from build123d import *

# Parameters (mm, degrees)
SKETCH1_W           = 70
SKETCH1_H           = 40
BOSS_EXTRUDE1_DEPTH = 1.7
SKETCH2_R           = 1
CUT_EXTRUDE1_DEPTH  = 1.7
SKETCH3_R           = 14
BOSS_EXTRUDE2_DEPTH = 30
SKETCH4_W           = 9.678505403
SKETCH4_H           = 8
BOSS_EXTRUDE3_DEPTH = 4
SKETCH5_W           = 6
SKETCH5_H           = 3
BOSS_EXTRUDE4_DEPTH = 4
SKETCH6_W           = 62
SKETCH6_H           = 32
BOSS_EXTRUDE5_DEPTH = 1
SKETCH7_W           = 35.794081109
SKETCH7_H           = 31.717706103
BOSS_EXTRUDE6_DEPTH = 1


with BuildPart() as part:
    # Sketch1 → Boss-Extrude1 (new body)
    with BuildSketch(Plane(origin=(0, 0, 0), x_dir=(1, 0, 0), z_dir=(0, 1, 0))):
        with Locations((35, 20)):
            Rectangle(SKETCH1_W, SKETCH1_H)
    extrude(amount=BOSS_EXTRUDE1_DEPTH)

    # Sketch2 → Cut-Extrude1 (cut)
    with BuildSketch(Plane(origin=(0, 1.7, 0), x_dir=(1, 0, 0), z_dir=(0, 1, 0))):
        with Locations(Location((67.8, 37.8, 0), (0, 0, 270))):
            Circle(SKETCH2_R)
        with Locations(Location((2.2, 37.8, 0), (0, 0, 270))):
            Circle(SKETCH2_R)
        with Locations(Location((2.2, 2.2, 0), (0, 0, 270))):
            Circle(SKETCH2_R)
        with Locations(Location((67.8, 2.2, 0), (0, 0, 270))):
            Circle(SKETCH2_R)
    extrude(amount=-CUT_EXTRUDE1_DEPTH, mode=Mode.SUBTRACT)

    # Sketch3 → Boss-Extrude2 (add)
    with BuildSketch(Plane(origin=(0, 1.7, 0), x_dir=(1, 0, 0), z_dir=(0, 1, 0))):
        with Locations(Location((15, 20, 0), (0, 0, 90))):
            Circle(SKETCH3_R)
    extrude(amount=BOSS_EXTRUDE2_DEPTH)

    # Sketch4 → Boss-Extrude3 (add)
    with BuildSketch(Plane(origin=(0, 1.7, 0), x_dir=(1, 0, 0), z_dir=(0, 1, 0))):
        with Locations((65.160747298, 27)):
            Rectangle(SKETCH4_W, SKETCH4_H)
    extrude(amount=BOSS_EXTRUDE3_DEPTH)

    # Sketch5 → Boss-Extrude4 (add)
    with BuildSketch(Plane(origin=(0, 1.7, 0), x_dir=(1, 0, 0), z_dir=(0, 1, 0))):
        with Locations((57, 16.5)):
            Rectangle(SKETCH5_W, SKETCH5_H)
    extrude(amount=BOSS_EXTRUDE4_DEPTH)

    # Sketch6 → Boss-Extrude5 (add)
    with BuildSketch(Plane.XZ):
        with Locations((35, -20)):
            Rectangle(SKETCH6_W, SKETCH6_H)
    extrude(amount=BOSS_EXTRUDE5_DEPTH)

    # Sketch7 → Boss-Extrude6 (add)
    with BuildSketch(Plane(origin=(0, 1.7, 0), x_dir=(1, 0, 0), z_dir=(0, 1, 0))):
        with Locations((48.346916126, 21.020495195)):
            Rectangle(SKETCH7_W, SKETCH7_H)
    extrude(amount=BOSS_EXTRUDE6_DEPTH)


solid = part.part
Could you check a few things on this model? Use its own coordinates, in mm. A direction names the side the tool comes from. Coordinates: 2 decimals unless noted, no trailing zeros. Write each loop counter-clockwise with the first axis right and the second up, starting at its lowest first coordinate (ties: lowest second). Pieces come first, ordered by that corner, then holes. Notation, with made-up numbers: (3.5, 71.5) - (10.5, 71.5) arc R36 cw to (10.5, 106.5) - close; hole circle Ø6 at (70, -16). An arc over 180 degrees is marked (long way). Put each result on its own line as item: value. Start each with the question number.
Q1. I want a section at B-B on x = 67.8. Write out the boundary of the cut face in (y, z), plus the area to 3 significant figures.
Q2. I want a section at D-D on z = -20. Write out the boundary of the cut face in (x, y), plus the area to 3 significant figures.
Q3. I want a section at A-A on z = -37.8. Write out the boundary of the cut face in (x, y).
Q4. I want a section at C-C on x = 15. Write out the boundary of the cut face in (y, z), plus the area to 3 significant figures.
Q5. Which directions (+Z, -Z, +X, -X, +Y, -Y) give clear straight access to the entire face, cutting with the end or side of a thin tool? Please do faces 4 (the flat face through (54, 4, -16)), 5 (the flat face through (57, 5.7, -17)), 6 (the flat face through (57, 4, -18)), 7 (the flat face through (57, 4, -15)).
Q6. I'm going to push flat-ended pins straight in: P1, Ø2.5, axis at x = 57.5, z = -16.5, coming from the +Y side; P2, Ø1.5, axis at y = 4.5, z = -16, coming from the -X side; P3, Ø2, axis at x = 59.5, y = 6, coming from the +Z side; P4, Ø4.5, axis at x = 63.5, y = 3.5, coming from the +Z side. Where does each tip first touch, or does it pass through?
Q7. Please list where these lines run through material, in increasing order: L1, parallel to X at y = 1.15, z = -37.8; L2, parallel to Z at x = 67.8, y = 0.8; L3, parallel to X at y = 1, z = -37.
Q8. Thinking about a two-plate mould opening in X: for faces 1 (the flat face through (35, 1, -40)), 2 (the cylindrical face through (2.2, 0.9, -38.8)), 3 (the flat face through (60, 4, -16)), which applies, pulls with the +X half, pulls with the -X half, needs draft (parallel to the pull), parting line crosses it, or undercut?
Checks:
1. outline: (0, -40) - (1.7, -40) - (1.7, -38.8) - (0, -38.8) - close; (0, -36.8) - (1.7, -36.8) - (1.7, -31) - (5.7, -31) - (5.7, -23) - (1.7, -23) - (1.7, -3.2) - (0, -3.2) - close; (0, -1.2) - (1.7, -1.2) - (1.7, 0) - (0, 0) - close
1. area: 93.2 mm²
2. outline: (0, 0) - (4, 0) - (4, -1) - (66, -1) - (66, 0) - (70, 0) - (70, 1.7) - (66.24, 1.7) - (66.24, 2.7) - (30.45, 2.7) - (30.45, 1.7) - (29, 1.7) - (29, 31.7) - (1, 31.7) - (1, 1.7) - (0, 1.7) - close
2. area: 1,060 mm²
3. outline: (0, 0) - (1.2, 0) - (1.2, 1.7) - (0, 1.7) - close; (3.2, 0) - (66.8, 0) - (66.8, 1.7) - (3.2, 1.7) - close; (68.8, 0) - (70, 0) - (70, 1.7) - (68.8, 1.7) - close
4. outline: (-1, -36) - (0, -36) - (0, -40) - (1.7, -40) - (1.7, -34) - (31.7, -34) - (31.7, -6) - (1.7, -6) - (1.7, 0) - (0, 0) - (0, -4) - (-1, -4) - close
4. area: 940 mm²
5. face 4: +Z, -Z, +Y
5. face 5: +Z, -Z, +X, +Y
5. face 6: -Z, +X, +Y
5. face 7: +Z, +X, +Y
6. P1: y = 5.7
6. P2: x = 1.38
6. P3: z = -15
6. P4: z = 0
7. L1: 0 to 1.2, 3.2 to 66.8, 68.8 to 70
7. L2: -40 to -38.8, -36.8 to -3.2, -1.2 to 0
7. L3: 0 to 1.6, 2.8 to 67.2, 68.4 to 70
8. face 1: needs draft
8. face 2: undercut
8. face 3: pulls with the +X half
